The model under review builds one solid part; all positions refer to its coordinate system, in mm. A direction names the side the tool comes from. Coordinates: 2 decimals unless noted, no trailing zeros. Write each loop counter-clockwise with the first axis right and the second up, starting at its lowest first coordinate (ties: lowest second). Pieces come first, ordered by that corner, then holes.
```python
from build123d import *

# Parameters (mm, degrees)
BASPROSKE_W         = 10
BASPROSKE_H         = 24.75
TOOTHCUT_DEPTH      = 37.402266413
TEETHCUTS_COUNT     = 20
TEETHCUTS_ANGLE     = 342
BORSKE_R            = 15
BORE_DEPTH          = 50.0000508
SKETCH1_R           = 15
BOSS_EXTRUDE1_DEPTH = 5
SKETCH2_R           = 7
CUT_EXTRUDE1_DEPTH  = 5
SKETCH3_R           = 1.25
CUT_EXTRUDE2_DEPTH  = 5


with BuildPart() as part:
    # BasProSke → Base-Revolve (revolve)
    with BuildSketch(Plane(origin=(0, 0, 0), x_dir=(1, 0, 0), z_dir=(0, 1, 0)), mode=Mode.PRIVATE) as base_revolve_sk:
        with Locations((5, 12.375)):
            Rectangle(BASPROSKE_W, BASPROSKE_H)
    revolve(base_revolve_sk.sketch.rotate(Axis((-10, 0, 0), (1, 0, 0)), 180), axis=Axis((-10, 0, 0), (1, 0, 0)))

    # TooCutSke → ToothCut (cut, through all)
    with BuildSketch(Plane(origin=(0, 0, 0), x_dir=(0, 0, -1), z_dir=(1, 0, 0))):
        with BuildLine():
            ThreePointArc((1.111948432, 19.655071939), (0, 19.6865), (-1.111948432, 19.655071939))
            ThreePointArc((-1.111948432, 19.655071939), (-1.832349961, 22.271720111), (-3.300041734, 24.55463642))
            ThreePointArc((-3.300041734, 24.55463642), (0, 24.7754), (3.300041734, 24.55463642))
            ThreePointArc((3.300041734, 24.55463642), (1.832349961, 22.271720111), (1.111948432, 19.655071939))
        make_face()
    toothcut = extrude(amount=TOOTHCUT_DEPTH, mode=Mode.SUBTRACT)

    # TeethCuts: ToothCut ×20 about axis
    teethcuts_axis = Axis((-10, 0, 0), (1, 0, 0))
    for i in range(1, TEETHCUTS_COUNT):
        add(toothcut.rotate(teethcuts_axis, i * TEETHCUTS_ANGLE / (TEETHCUTS_COUNT - 1)), mode=Mode.SUBTRACT)

    # BorSke → Bore (cut, symmetric)
    with BuildSketch(Plane(origin=(0, 0, 0), x_dir=(0, 0, -1), z_dir=(1, 0, 0))):
        with Locations(Location((0, 0, 0), (0, 0, 180))):
            Circle(BORSKE_R)
    extrude(amount=BORE_DEPTH, both=True, mode=Mode.SUBTRACT)

    # Sketch1 → Boss-Extrude1 (add)
    with BuildSketch(Plane(origin=(10, 0, 0), x_dir=(0, 0, -1), z_dir=(1, 0, 0))):
        Circle(SKETCH1_R)
    extrude(amount=-BOSS_EXTRUDE1_DEPTH)

    # Sketch2 → Cut-Extrude1 (cut)
    with BuildSketch(Plane(origin=(10, 0, 0), x_dir=(0, 0, -1), z_dir=(1, 0, 0))):
        Circle(SKETCH2_R)
    extrude(amount=-CUT_EXTRUDE1_DEPTH, mode=Mode.SUBTRACT)

    # Sketch3 → Cut-Extrude2 (cut)
    with BuildSketch(Plane(origin=(10, 0, 0), x_dir=(0, 0, -1), z_dir=(1, 0, 0))):
        with Locations((0, 12)):
            Circle(SKETCH3_R)
        with Locations((8.485281374, 8.485281374)):
            Circle(SKETCH3_R)
        with Locations((12, 0)):
            Circle(SKETCH3_R)
        with Locations((8.485281374, -8.485281374)):
            Circle(SKETCH3_R)
        with Locations((0, -12)):
            Circle(SKETCH3_R)
        with Locations((-8.485281374, -8.485281374)):
            Circle(SKETCH3_R)
        with Locations((-12, 0)):
            Circle(SKETCH3_R)
        with Locations((-8.485281374, 8.485281374)):
            Circle(SKETCH3_R)
    extrude(amount=-CUT_EXTRUDE2_DEPTH, mode=Mode.SUBTRACT)


solid = part.part
```
Item 1: Mouldability with a two-part tool opening along Y and no side actions: class faces 4 (the face through (7.535, -2.681, -6.466)), 5 (the face through (4.93, -22.29, 1.84)), 6 (the face through (5.07, 24.447, 3.863)) as pulls with the +Y half, pulls with the -Y half, needs draft (parallel to the pull), parting line crosses it, or undercut.
Solved:
face 4: undercut
face 5: pulls with the -Y half
face 6: pulls with the +Y half
Item 2: Take a section at B-B, the plane y = -20.5. Write out the cut boundary in (x, z), plus the area to 3 significant figures.
Solved:
outline: (0, -11.79) - (10, -11.79) - (10, -8.52) - (0, -8.52) - close; (0, -5.19) - (10, -5.19) - (10, -1.25) - (0, -1.25) - close; (0, 1.25) - (10, 1.25) - (10, 5.19) - (0, 5.19) - close; (0, 8.52) - (10, 8.52) - (10, 11.79) - (0, 11.79) - close
area: 144 mm2
Item 3: Machinability: for faces 1 (the face through (4.93, 5.137, -21.77)), 2 (the face through (4.9, -22.2, -1.8)), 3 (the face through (4.93, -14.59, -16.95)), which of the approach directions +Z, -Z, +X, -X, +Y, -Y give a long, thin tool a straight path to every point of the face, cutting with its end or side? Answer none if there is none.
Solved:
face 1: +X, -X
face 2: +X, -X, -Y
face 3: -Z, +X, -X
Item 4: Take a section at A-A, the plane z = 0. Write out the cut boundary in (x, y), plus the area to 3 significant figures.
Solved:
outline: (0, -19.69) - (10, -19.69) - (10, -13.25) - (5, -13.25) - (5, -15) - (0, -15) - close; (0, 15) - (5, 15) - (5, 13.25) - (10, 13.25) - (10, 19.69) - (0, 19.69) - close; (5, -10.75) - (10, -10.75) - (10, -7) - (5, -7) - close; (5, 7) - (10, 7) - (10, 10.75) - (5, 10.75) - close
area: 149 mm2
Item 5: To check wall thickness, follow line 1 along Y through (x, z) = (9.25, -15.5); line 2 along Z through (x, y) = (6.25, 20.5); line 3 along Y through (x, z) = (7, -21). State the ranges of each line that lie inside material, in increasing order.
Solved:
line 1: y = -17.41 to -12.69, -12.14 to 12.14, 12.69 to 17.41
line 2: z = -11.79 to -8.52, -5.19 to -1.25, 1.25 to 5.19, 8.52 to 11.79
line 3: y = -11.8 to -8.99, -5.19 to -1.38, 1.38 to 5.19, 8.99 to 11.8
Item 6: For pin 1 (2 mm diameter, centred on x = 5.5, z = 15.5, fed in from +Y); pin 2 (9 mm diameter, centred on y = 1, z = -2.5, fed in from -X); pin 3 (3 mm diameter, centred on x = 9, y = 0.5, fed in from +Z); pin 4 (8.5 mm diameter, centred on y = 0, z = 0, fed in from -X), all flat-tipped, find the tip position at first contact; note any pin that passes through.
Solved:
pin 1: stops at y = 17.77
pin 2: stops at x = 5
pin 3: stops at z = 22.63
pin 4: passes through
